CAD build for the part. Positions are in the model's coordinates, mm. Face numbers are marked on the shaded views. A direction names the side the tool comes from. Coordinates: 2 decimals unless noted, no trailing zeros. Loops run counter-clockwise (first coordinate to the right, second up) from the corner with the lowest first, then second, coordinate; pieces in that order, holes last. Notation, with made-up numbers: (29.5, 29.5) -> (66.5, 29.5) arc R25 cw to (66.5, 46.5) -> close; hole circle Ø5 at (23.25, -26). An arc over 180 degrees is marked (long way). Answer as CSV lines item,"result". Start each with the question number.
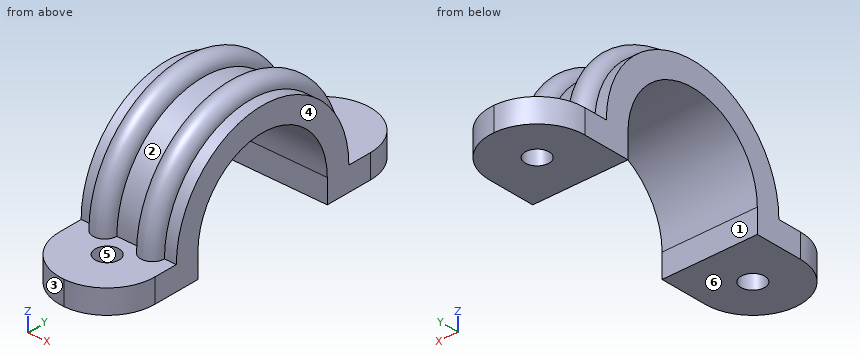
Solid Edge part; units mm, degrees
sketch "Sketch1" plane through (0, 0, 0) normal (0, 0, 1) x (1, 0, 0)
  line L0 (-10, 15) -> (10, 15)
  line L1 (10, 15) -> (10, 35)
  line L2 (10, 35) -> (-10, 35)
  line L3 (-10, 35) -> (-10, 15)
  dimension "D1" = 10
  dimension "D2" = 10
extrude "Protrusion1" add sketch "Sketch1" along normal blind 5
hole "Hole_1" at (0, 25, 5) direction (0, 0, -1) diameter 5 end up to next
fillet "Round_1" radius 10 2 edges at (10, 35, 2.5) (-10, 35, 2.5)
mirror "Mirror1" about plane through (0, 0, 0) normal (0, 1, 0) of "Protrusion1", "Hole_1"
fillet "Round1" radius 10 2 edges at (10, -35, 2.5) (-10, -35, 2.5)
sketch "Sketch2" plane through (0, 40, 5) normal (0, 0, 1) x (1, 0, 0)
  line L0 (-10, -25) -> (10, -25)
  line L1 (10, -25) -> (10, -20)
  line L2 (10, -20) -> (7.5, -20)
  arc A0 (2.5, -20) -> (7.5, -20) centre (5, -20) cw
  line L3 (2.5, -20) -> (-2.5, -20)
  arc A1 (-7.5, -20) -> (-2.5, -20) centre (-5, -20) cw
  line L4 (-7.5, -20) -> (-10, -20)
  line L5 (-10, -20) -> (-10, -25)
  dimension "D1" = 10
revolve "RevolvedProtrusion_1" add sketch "Sketch2" angle 180 about axis through (0, 0, 5) along (1, 0, 0)
Item 1: Which spindle directions (+Z, -Z, +X, -X, +Y, -Y) get a long thin tool onto all of the face, cutting with end or side? Do the marked faces 1, 2 and 3. Say none if no direction does.
Item 2: Saw through at A-A (y = 0). Write the cut outline in (x, z), plus the area to 3 significant figures.
Item 3: Wall check: probe 1 along Y at (x, z) = (0, 3.8); probe 2 along Z at (x, y) = (-2, -21.5); probe 3 along X at (y, z) = (17, 18.5). Give the ranges that are in metal, low to high.
Item 4: Saw through at B-B (x = -1.75). Write the cut outline in (y, z), plus the area to 3 significant figures.
Item 5: Saw through at C-C (x = 3.5). Write the cut outline in (y, z).
Item 6: Saw through at D-D (x = 8.25). Write the cut outline in (y, z), plus the area to 3 significant figures.
Item 7: Two-plate mould, pull along X, no slides. Class the marked faces 4, 5 and 6: pulls with the +X half, pulls with the -X half, needs draft (parallel to the pull), parting line crosses it, or undercut.
Item 8: Flat gauge pins, fed straight in: pin 1 Ø7.5 at (x, y) = (-3.5, 27) entering from +Z; pin 2 Ø1.5 at (x, y) = (0.5, 0) entering from -Z; pin 3 Ø1 at (x, z) = (0.5, 10.5) entering from -Y. Where does each tip first touch, or does it go through?
Geometry check:
1,face 1,"-Z, +X, -X"
1,face 2,"+Z"
1,face 3,"+Z, -Z, -X, -Y"
2,outline,"(-10, 20) -> (10, 20) -> (10, 25) -> (7.5, 25) arc R2.5 ccw to (2.5, 25) -> (-2.5, 25) arc R2.5 ccw to (-7.5, 25) -> (-10, 25) -> close"
2,area,"120 mm2"
3,probe 1,"-35 to -27.5, -22.5 to -15, 15 to 22.5, 27.5 to 35"
3,probe 2,"0 to 5"
3,probe 3,"-6.83 to -3.17, 3.17 to 6.83"
4,outline,"(-34.85, 0) -> (-26.79, 0) -> (-26.79, 5) -> (-34.85, 5) -> close; (-23.21, 0) -> (-15, 0) -> (-15, 5) arc R15 cw to (15, 5) -> (15, 0) -> (23.21, 0) -> (23.21, 5) -> (20, 5) arc R20 ccw to (-20, 5) -> (-23.21, 5) -> close; (26.79, 0) -> (34.85, 0) -> (34.85, 5) -> (26.79, 5) -> close"
4,area,"438 mm2"
5,outline,"(-34.37, 0) -> (-15, 0) -> (-15, 5) arc R15 cw to (15, 5) -> (15, 0) -> (34.37, 0) -> (34.37, 5) -> (22, 5) arc R22 ccw to (-22, 5) -> (-34.37, 5) -> close"
6,outline,"(-30.65, 0) -> (-15, 0) -> (-15, 5) arc R15 cw to (15, 5) -> (15, 0) -> (30.65, 0) -> (30.65, 5) -> (20, 5) arc R20 ccw to (-20, 5) -> (-30.65, 5) -> close"
6,area,"431 mm2"
7,face 4,"pulls with the +X half"
7,face 5,"undercut"
7,face 6,"needs draft"
8,pin 1,"z = 5"
8,pin 2,"z = 19.98"
8,pin 3,"y = -19.36"
